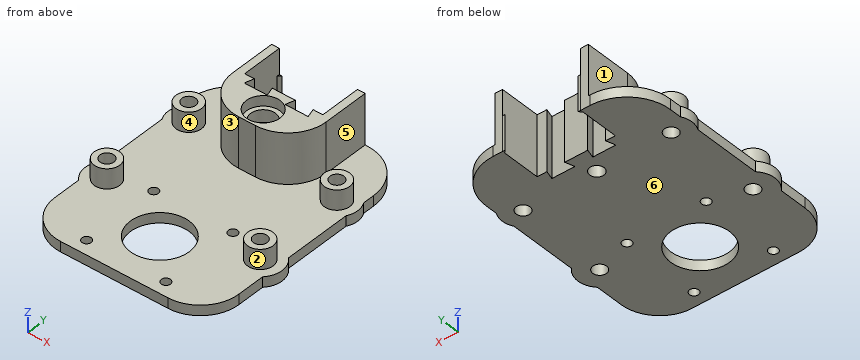
```python
from build123d import *

# Parameters (mm, degrees)
SKETCH_1_R           = 2.8
SKETCH_1_R_2         = 2.7
SKETCH_1_R_3         = 1.8
SKETCH_1_R_4         = 11.5
EXTRUDE_1_DEPTH      = 4
EXTRUDE_START        = 4
SKETCH_1_4_R         = 2.8
EXTRUDE_3_DEPTH      = 19.6
SKETCH_9_R           = 5
SKETCH_9_R_2         = 2.7
EXTRUDE_4_DEPTH      = 7.7
FILLET_1_R           = 15
SKETCH_12_R          = 6.6
CUT_EXTRUDE_12_DEPTH = 4
CUT_EXTRUDE_START    = -8.8
SKETCH_12_5_R        = 4.849742261
SKETCH_12_5_R_2      = 2.8
CUT_EXTRUDE_13_DEPTH = 4.8
CUT_EXTRUDE_14_REACH = 72.202
CUT_EXTRUDE_15_DEPTH = 10


with BuildPart() as part:
    # 草图1 → 凸台-拉伸1 (new body)
    with BuildSketch(Plane.XY):
        with BuildLine():
            Line((-11.5, 37.75), (-15.3, 37.75))
            Line((-15.3, 37.75), (-15.3, 52.749))
            Line((-15.3, 52.749), (-14.3, 53.749))
            Line((-14.3, 53.749), (-15.3, 53.749))
            Line((-15.3, 53.749), (-15.3, 53.75))
            Line((-15.3, 53.75), (-19, 53.75))
            ThreePointArc((-19, 53.75), (-31.02081528, 48.77081528), (-36, 36.75))
            Line((-36, 36.75), (-36, 32.175536774))
            ThreePointArc((-36, 32.175536774), (-37.1, 28.1), (-36, 24.024463226))
            Line((-36, 24.024463226), (-36, -2.479202711))
            ThreePointArc((-36, -2.479202711), (-38.5, -8.5), (-36, -14.520797289))
            Line((-36, -14.520797289), (-36, -25.5))
            ThreePointArc((-36, -25.5), (-31.606601718, -36.106601718), (-21, -40.5))
            Line((-21, -40.5), (21, -40.5))
            ThreePointArc((21, -40.5), (31.606601718, -36.106601718), (36, -25.5))
            Line((36, -25.5), (36, -14.520797289))
            ThreePointArc((36, -14.520797289), (38.5, -8.5), (36, -2.479202711))
            Line((36, -2.479202711), (36, 24.024463226))
            ThreePointArc((36, 24.024463226), (37.1, 28.1), (36, 32.175536774))
            Line((36, 32.175536774), (36, 36.75))
            ThreePointArc((36, 36.75), (31.02081528, 48.77081528), (19, 53.75))
            Line((19, 53.75), (15.3, 53.75))
            Line((15.3, 53.75), (15.3, 53.749))
            Line((15.3, 53.749), (14.3, 53.749))
            Line((14.3, 53.749), (15.3, 52.749))
            Line((15.3, 52.749), (15.3, 37.75))
            Line((15.3, 37.75), (11.5, 37.75))
            Line((11.5, 37.75), (11.5, 34.25))
            Line((11.5, 34.25), (4.5, 34.25))
            Line((4.5, 34.25), (4.5, 37.75))
            Line((4.5, 37.75), (-4.5, 37.75))
            Line((-4.5, 37.75), (-4.5, 34.25))
            Line((-4.5, 34.25), (-11.5, 34.25))
            Line((-11.5, 34.25), (-11.5, 37.75))
        make_face()
        with Locations((0, 28.25)):
            Circle(SKETCH_1_R, mode=Mode.SUBTRACT)
        with Locations((-29, 28.1)):
            Circle(SKETCH_1_R_2, mode=Mode.SUBTRACT)
        with Locations((-30, -8.5)):
            Circle(SKETCH_1_R_2, mode=Mode.SUBTRACT)
        with Locations((29, 28.1)):
            Circle(SKETCH_1_R_2, mode=Mode.SUBTRACT)
        with Locations((30, -8.5)):
            Circle(SKETCH_1_R_2, mode=Mode.SUBTRACT)
        with Locations((15.5, -4)):
            Circle(SKETCH_1_R_3, mode=Mode.SUBTRACT)
        with Locations((0, -19.5)):
            Circle(SKETCH_1_R_4, mode=Mode.SUBTRACT)
        with Locations((15.5, -35)):
            Circle(SKETCH_1_R_3, mode=Mode.SUBTRACT)
        with Locations((-15.5, -35)):
            Circle(SKETCH_1_R_3, mode=Mode.SUBTRACT)
        with Locations((-15.5, -4)):
            Circle(SKETCH_1_R_3, mode=Mode.SUBTRACT)
    extrude(amount=EXTRUDE_1_DEPTH)

    # 草图1<4> → 凸台-拉伸3 (add)
    with BuildSketch(Plane.XY.offset(EXTRUDE_START)):
        Polygon((-11.5, 37.75), (-15.3, 37.75), (-15.3, 52.749), (-14.3, 53.749), (-15.3, 53.749), (-15.3, 53.75), (-18.3, 53.75), (-18.3, 20.75), (18.3, 20.75), (18.3, 53.75), (15.3, 53.75), (15.3, 53.749), (14.3, 53.749), (15.3, 52.749), (15.3, 37.75), (11.5, 37.75), (11.5, 34.25), (4.5, 34.25), (4.5, 37.75), (-4.5, 37.75), (-4.5, 34.25), (-11.5, 34.25), align=None)
        with Locations((0, 28.25)):
            Circle(SKETCH_1_4_R, mode=Mode.SUBTRACT)
    extrude(amount=EXTRUDE_3_DEPTH)

    # 草图9 → 凸台-拉伸4 (add)
    # profile 1 of 4: a face of its own
    with BuildSketch(Plane.XY.offset(4)):
        with Locations(Location((-29, 28.1, 0), (0, 0, 180))):
            Circle(SKETCH_9_R)
        with Locations((-29, 28.1)):
            Circle(SKETCH_9_R_2, mode=Mode.SUBTRACT)
    # profile 2 of 4: a face of its own
    with BuildSketch(Plane.XY.offset(4)):
        with Locations(Location((-30, -8.5, 0), (0, 0, 180))):
            Circle(SKETCH_9_R)
        with Locations((-30, -8.5)):
            Circle(SKETCH_9_R_2, mode=Mode.SUBTRACT)
    # profile 3 of 4: a face of its own
    with BuildSketch(Plane.XY.offset(4)):
        with Locations(Location((30, -8.5, 0), (0, 0, 180))):
            Circle(SKETCH_9_R)
        with Locations(Location((30, -8.5, 0), (0, 0, 180))):
            Circle(SKETCH_9_R_2, mode=Mode.SUBTRACT)
    # profile 4 of 4: a face of its own
    with BuildSketch(Plane.XY.offset(4)):
        with Locations(Location((29, 28.1, 0), (0, 0, 180))):
            Circle(SKETCH_9_R)
        with Locations(Location((29, 28.1, 0), (0, 0, 180))):
            Circle(SKETCH_9_R_2, mode=Mode.SUBTRACT)
    extrude(amount=EXTRUDE_4_DEPTH)

    # 圆角1
    fillet_1_edges = [part.edges().sort_by_distance(p)[0] for p in [
        (-18.3, 20.75, 13.8),
        (18.3, 20.75, 13.8),
    ]]
    fillet(fillet_1_edges, radius=FILLET_1_R)

    # 草图12 → 切除-拉伸12 (cut)
    with BuildSketch(Plane.XY.offset(23.6)):
        with Locations((0, 28.25)):
            Circle(SKETCH_12_R)
    extrude(amount=-CUT_EXTRUDE_12_DEPTH, mode=Mode.SUBTRACT)

    # 草图12<5> → 切除-拉伸13 (cut)
    with BuildSketch(Plane.XY.offset(23.6).offset(CUT_EXTRUDE_START)):
        with Locations((0, 28.25)):
            Circle(SKETCH_12_5_R)
        with Locations((0, 28.25)):
            Circle(SKETCH_12_5_R_2, mode=Mode.SUBTRACT)
    extrude(amount=CUT_EXTRUDE_13_DEPTH, mode=Mode.SUBTRACT)

    # 草图13 → 切除-拉伸14 (cut, up to next)
    with BuildSketch(Plane.XY.offset(23.6), mode=Mode.PRIVATE) as cut_extrude_14_sk1:
        Polygon((-4.5, 37.75), (-3.5, 34.25), (-4.5, 34.25), align=None)
    cut_extrude_14_tool1 = extrude(cut_extrude_14_sk1.sketch, amount=-CUT_EXTRUDE_14_REACH, mode=Mode.PRIVATE) & part.part
    # 草图13 → 切除-拉伸14 (cut, up to next)
    with BuildSketch(Plane.XY.offset(23.6), mode=Mode.PRIVATE) as cut_extrude_14_sk2:
        Polygon((-11.5, 34.25), (-11.5, 37.75), (-12.5, 34.25), align=None)
    cut_extrude_14_tool2 = extrude(cut_extrude_14_sk2.sketch, amount=-CUT_EXTRUDE_14_REACH, mode=Mode.PRIVATE) & part.part
    # 草图13 → 切除-拉伸14 (cut, up to next)
    with BuildSketch(Plane.XY.offset(23.6), mode=Mode.PRIVATE) as cut_extrude_14_sk3:
        Polygon((11.5, 37.75), (12.5, 34.25), (11.5, 34.25), align=None)
    cut_extrude_14_tool3 = extrude(cut_extrude_14_sk3.sketch, amount=-CUT_EXTRUDE_14_REACH, mode=Mode.PRIVATE) & part.part
    # 草图13 → 切除-拉伸14 (cut, up to next)
    with BuildSketch(Plane.XY.offset(23.6), mode=Mode.PRIVATE) as cut_extrude_14_sk4:
        Polygon((4.5, 34.25), (4.5, 37.75), (3.5, 34.25), align=None)
    cut_extrude_14_tool4 = extrude(cut_extrude_14_sk4.sketch, amount=-CUT_EXTRUDE_14_REACH, mode=Mode.PRIVATE) & part.part
    add(cut_extrude_14_tool1.solids().sort_by_distance((-4.166667, 35.416667, 23.6))[0], mode=Mode.SUBTRACT)
    add(cut_extrude_14_tool2.solids().sort_by_distance((-11.833333, 35.416667, 23.6))[0], mode=Mode.SUBTRACT)
    add(cut_extrude_14_tool3.solids().sort_by_distance((11.833333, 35.416667, 23.6))[0], mode=Mode.SUBTRACT)
    add(cut_extrude_14_tool4.solids().sort_by_distance((4.166667, 35.416667, 23.6))[0], mode=Mode.SUBTRACT)

    # 草图14 → 切除-拉伸15 (cut)
    with BuildSketch(Plane.XY.offset(23.6)):
        Polygon((-15.3, 53.749), (-15.3, 52.749), (-14.3, 53.749), align=None)
        Polygon((14.3, 53.749), (15.3, 52.749), (15.3, 53.749), align=None)
    extrude(amount=-CUT_EXTRUDE_15_DEPTH, mode=Mode.SUBTRACT)


solid = part.part
```
Geometry: final body of the model. Coordinates: model frame, mm. Face numbers are marked on the shaded views. A direction names the side the tool comes from. Coordinates: 2 decimals unless noted, no trailing zeros. Loops run counter-clockwise (first coordinate to the right, second up) from the corner with the lowest first, then second, coordinate; pieces in that order, holes last. Notation, with made-up numbers: M -23.75,15.25 L -16.75,15.25 A26 ccw -16.75,51.25 Z; hole C 21,38 d6. An arc over 180 degrees is marked long. Put each result on its own line as item: value.
(1) Cut plane B-B on y = -16.5. Return the cut outline in (x, z).
Answer sheet:
outline: M -36,0 L -11.1,0 L -11.1,4 L -36,4 Z; M 11.1,0 L 36,0 L 36,4 L 11.1,4 Z
(2) Cut plane A-A on z = 10.25. State how many separate pieces and enclosed holes the cut face has, then the cut area to 3 significant figures.
Answer sheet:
separate pieces: 5
enclosed holes: 5
area: 765 mm^2
(3) Access query for the marked faces 1, 2 and 3. Directions: +Z, -Z, +X, -X, +Y, -Y. A direction counts if a zero-diameter tool reaches every point of the face in a straight line with its end or side. Return the directions, or none.
Answer sheet:
face 1: +Z, -X, +Y, -Y
face 2: +Z
face 3: +Z, -Y
(4) First-contact query: pin 1 (1.1 mm diameter, centred on x = 14.5, y = 53.5, fed in from +Z); pin 2 (8 mm diameter, centred on y = 48, z = 17, fed in from +X); pin 3 (6 mm diameter, centred on y = 28, z = 18.5, fed in from +X). Flat tips, straight axial feed; report the tip coordinate or a pass-through.
Answer sheet:
pin 1: stops at z = 13.6
pin 2: stops at x = 18.3
pin 3: stops at x = 17.53
(5) Cut plane D-D on z = 22. Return the cut outline in (x, y).
Answer sheet:
outline: M -18.3,35.75 A15 ccw -3.3,20.75 L 3.3,20.75 A15 ccw 18.3,35.75 L 18.3,53.75 L 15.3,53.75 L 15.3,37.75 L 11.5,37.75 L 12.5,34.25 L 3.5,34.25 L 4.5,37.75 L -4.5,37.75 L -3.5,34.25 L -12.5,34.25 L -11.5,37.75 L -15.3,37.75 L -15.3,53.75 L -18.3,53.75 Z; hole C 0,28.25 d13.2
(6) Cut plane C-C on x = -9.5. Return the cut outline in (y, z), then the cut area to 3 significant figures.
Answer sheet:
outline: M -40.5,0 L -25.98,0 L -25.98,4 L -40.5,4 Z; M -13.02,0 L 34.25,0 L 34.25,23.6 L 22.09,23.6 L 22.09,4 L -13.02,4 Z
area: 485 mm^2
(7) Material intervals for probe 1 along Y at (x, z) = (15.5, 2.6); probe 2 along Y at (x, z) = (0, 8.5); probe 3 along Y at (x, z) = (14, 2.25), sorted ascending.
Answer sheet:
probe 1: y = -40.5 to -36.8, -33.2 to -5.8, -2.2 to 53.75
probe 2: y = 20.75 to 25.45, 31.05 to 37.75
probe 3: y = -40.5 to -35.99, -34.01 to -4.99, -3.01 to 37.75
(8) Draft query along X for the marked faces 4, 5 and 6. Return one class per face: pulls with the +X half, pulls with the -X half, needs draft (parallel to the pull), parting line crosses it, or undercut.
Answer sheet:
face 4: undercut
face 5: pulls with the +X half
face 6: needs draft
